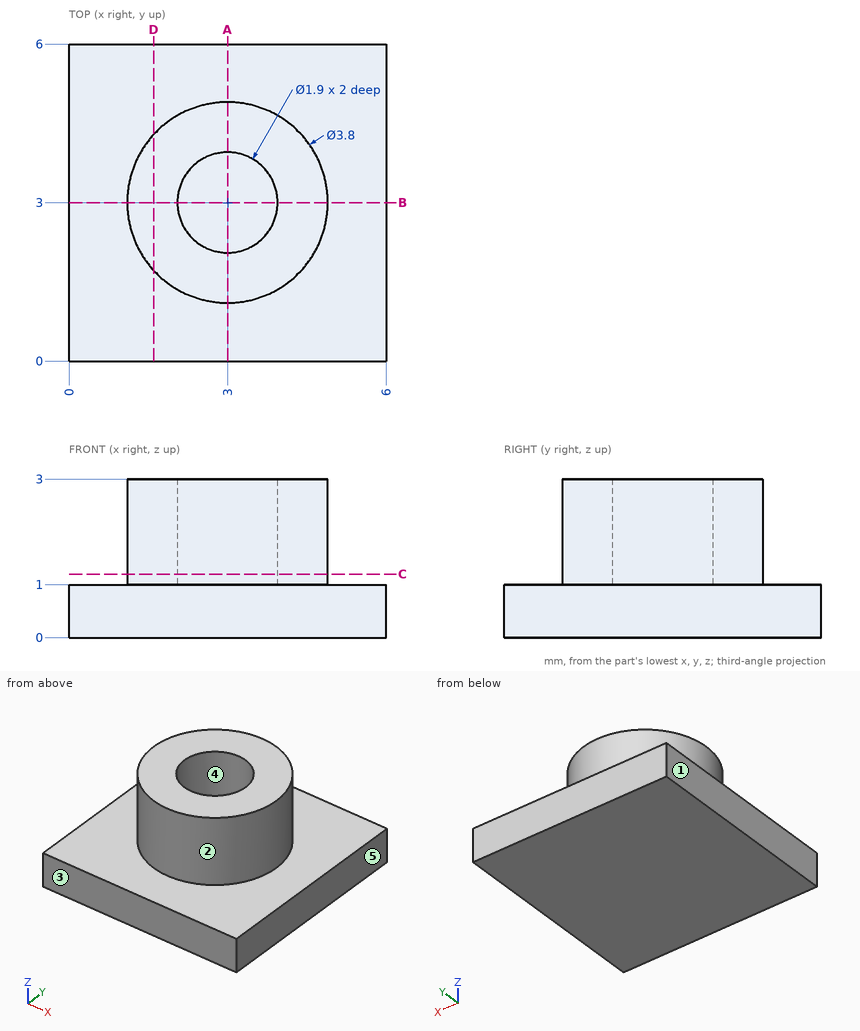
Geometry check sheet. Reference: drawing and pictorial views, mm from the part's lowest x, y, z. A direction names the side the tool comes from. Give positions to 0.01 mm unless a question says otherwise; leave off trailing zeros. Write each loop counter-clockwise with the first axis right and the second up, starting at its lowest first coordinate (ties: lowest second). Pieces come first, ordered by that corner, then holes. Notation, with made-up numbers: (-30, 72.5) -> (12, 72.5) arc R31 cw to (12, 100.5) -> close; hole circle Ø4 at (71, 5). An arc over 180 degrees is marked (long way). One line per item, written item: value. Start each with the question number.
Item 1: Section check D-D on x = 1.6. Record the cut outline in (y, z).
Item 2: Draft check along Y on the marked faces 3, 4 and 5. Enter one of: +Y half, -Y half, draft (parallel to the pull), parting line (faces both ways), or undercut.
Item 3: Section check C-C on z = 1.2. Record the cut outline in (x, y), then the cut area to 3 significant figures.
Item 4: Section check A-A on x = 3. Record the cut outline in (y, z).
Item 5: Gauge pin test, flat end, axial feed: pin 1 (1 mm diameter, centred on x = 1.5, z = 2, fed in from -Y). Record the tip position at first contact, or that the pin passes through.
Item 6: Tool access check on the marked faces 1 and 2. Record the directions out of +Z, -Z, +X, -X, +Y, -Y that give a thin tool (end or side, any length) a straight path to the whole face; none if there is none.
Item 7: Material ranges on probe 1 along Y at (x, z) = (3, 2.7); probe 2 along Z at (x, y) = (0.3, 0.9); probe 3 along Y at (x, z) = (3.75, 1.85), recorded low to high. Write a range as from..to.
Results list:
1. outline: (0, 0) -> (6, 0) -> (6, 1) -> (4.28, 1) -> (4.28, 3) -> (1.72, 3) -> (1.72, 1) -> (0, 1) -> close
2. face 3: -Y half
2. face 4: undercut
2. face 5: draft
3. outline: circle Ø3.8 at (3, 3); hole circle Ø1.9 at (3, 3)
3. area: 8.51 mm²
4. outline: (0, 0) -> (6, 0) -> (6, 1) -> (4.9, 1) -> (4.9, 3) -> (3.95, 3) -> (3.95, 1) -> (2.05, 1) -> (2.05, 3) -> (1.1, 3) -> (1.1, 1) -> (0, 1) -> close
5. pin 1: y = 1.38
6. face 1: +Z, -Z, -X, +Y, -Y
6. face 2: +Z
7. probe 1: 1.1..2.05, 3.95..4.9
7. probe 2: 0..1
7. probe 3: 1.25..2.42, 3.58..4.75
